Source: CAD feature listing. Evaluate the final solid. Frame: model axes, mm. Face numbers are marked on the shaded views. Round coordinates to 2 decimals unless told otherwise and drop trailing zeros. Loops run counter-clockwise (first coordinate to the right, second up) from the corner with the lowest first, then second, coordinate; pieces in that order, holes last. Notation, with made-up numbers: (-5, 47) -> (48, 47) arc R22 ccw to (48, 66) -> close; hole circle Ø9 at (55.25, 73.25). An arc over 180 degrees is marked (long way). Write item = value, one per line.
from build123d import *

# Parameters (mm, degrees)
SKETCH1_W                        = 12.7
SKETCH1_H                        = 38.1
EXTRUDE1_DEPTH                   = 76.2
F_3_8_16_TAPPED_HOLE1_D          = 7.9375
F_3_8_16_TAPPED_HOLE1_DEPTH      = 12.7
F_3_8_0_375_DIAMETER_HOLE1_D     = 9.525
F_3_8_0_375_DIAMETER_HOLE1_DEPTH = 12.7
SKETCH6_R                        = 12.827
EXTRUDE2_DEPTH                   = 3.175


with BuildPart() as part:
    # Sketch1 → Extrude1 (new body, symmetric)
    with BuildSketch(Plane.XY):
        Rectangle(SKETCH1_W, SKETCH1_H)
    extrude(amount=EXTRUDE1_DEPTH, both=True)

    # 3/8-16 Tapped Hole1
    with Locations(Plane(origin=(6.35, 0, 0), x_dir=(0, 0, -1), z_dir=(1, 0, 0))):
        with Locations((-60.325, 0), (60.325, 0)):
            Hole(F_3_8_16_TAPPED_HOLE1_D / 2, depth=F_3_8_16_TAPPED_HOLE1_DEPTH)

    # 3/8 (0.375) Diameter Hole1
    with Locations(Plane(origin=(6.35, 0, 0), x_dir=(0, 0, -1), z_dir=(1, 0, 0))):
        with Locations((0, 0)):
            Hole(F_3_8_0_375_DIAMETER_HOLE1_D / 2, depth=F_3_8_0_375_DIAMETER_HOLE1_DEPTH)

    # Sketch6 → Extrude2 (cut)
    with BuildSketch(Plane.ZY.offset(6.35)):
        Circle(SKETCH6_R)
    extrude(amount=-EXTRUDE2_DEPTH, mode=Mode.SUBTRACT)


solid = part.part
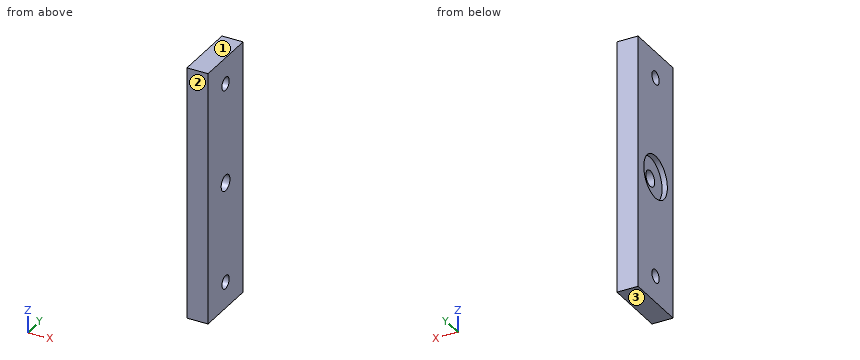
1. Section query D-D (y = 9). Return the cut outline in (x, z) (3 decimals).
Evaluation:
outline = (-6.35, -76.2) -> (6.35, -76.2) -> (6.35, 76.2) -> (-6.35, 76.2) -> (-6.35, 9.14) -> (-3.175, 9.14) -> (-3.175, -9.14) -> (-6.35, -9.14) -> close
2. Mould query, pull axis Z, two halves, no side actions, for the marked faces 1, 2 and 3. Classes: released by +Z, released by -Z, zero draft, split by the parting line, or undercut.
Evaluation:
face_1 = released by +Z
face_2 = zero draft
face_3 = released by -Z
3. Contact query for flat-ended pins moving along their axis: pin 1 Ø7.5 at (y, z) = (0, 0) entering from +X; pin 2 Ø20.5 at (y, z) = (0, 0) entering from -X (3 decimals). Output: stop coordinate, or through.
Evaluation:
pin_1 = through
pin_2 = -3.175
4. Line query: probe 1 along Y at (x, z) = (-0.75, 0); probe 2 along X at (y, z) = (-7, -4) (3 decimals); probe 3 along Z at (x, y) = (-3, -4). Output: solid intervals per line, ascending. Write a range as from..to.
Evaluation:
probe_1 = -19.05..-4.76, 4.76..19.05
probe_2 = -3.175..6.35
probe_3 = -76.2..-2.58, 2.58..76.2
5. Section query B-B (x = -4.75). Give the number of separate pieces and of enclosed holes in the cut face, then the cut area to 3 significant figures.
Evaluation:
separate_pieces = 1
enclosed_holes = 3
area = 5,190 mm²
